from build123d import *

# Parameters (mm, degrees)
PAD_DEPTH            = 6.5
POCKET_DEPTH         = 6
SKETCH002_R          = 13.5
POCKET001_DEPTH      = 1
SKETCH003_W          = 5.4
SKETCH003_H          = 6.5
PAD001_DEPTH         = 3.5
POCKET002_DEPTH      = 10
SKETCH010_W          = 3.95
SKETCH010_H          = 6.5
PAD002_DEPTH         = 3.5
POCKET005_DEPTH      = 10
SKETCH014_R          = 20.45
SKETCH014_R_2        = 19.85
POCKET008_DEPTH      = 0.3
SKETCH015_R          = 2.2
SKETCH015_R_2        = 1.025
PAD003_DEPTH         = 2
POCKET009_DEPTH      = 4
POCKET010_DEPTH      = 4
PAD004_DEPTH         = 4
POCKET013_DEPTH      = 12.151
POCKET013_DEPTH_BACK = 36.251
SKETCH022_R          = 0.6
POCKET014_DEPTH      = 2
SKETCH023_R          = 0.6
POCKET015_DEPTH      = 2


with BuildPart() as part:
    # Sketch → Pad (new body)
    with BuildSketch(Plane.XY):
        with BuildLine():
            Line((-22.5019915649, 16), (-22.5019915649, -16))
            Line((-22.5019915649, -16), (-16.2858834578, -17.9))
            ThreePointArc((-16.2858834578, -17.9), (-0.4552796053, -24.1957169863), (15.6009615088, -18.5))
            Line((15.6009615088, -18.5), (24.5395016581, -17.45))
            Line((24.5395016581, 17.45), (24.5395016581, -17.45))
            Line((15.6009615088, 18.5), (24.5395016581, 17.45))
            ThreePointArc((15.6009615088, 18.5), (-0.4552796053, 24.1957169863), (-16.2858834578, 17.9))
            Line((-22.5019915649, 16), (-16.2858834578, 17.9))
        make_face()
    extrude(amount=PAD_DEPTH)

    # Sketch001 → Pocket (cut)
    with BuildSketch(Plane.XY):
        with BuildLine():
            Line((-14.8539557021, 16.9), (-21.2122180433, 15.55))
            Line((-21.2122180433, 15.55), (-21.2122180433, -15.55))
            Line((-21.2122180433, -15.55), (-14.8539557021, -16.9))
            ThreePointArc((-14.8539557021, -16.9), (-0.0760301383, -22.4998715423), (14.739402973, -17))
            Line((14.739402973, -17), (23.6191552218, -16.4))
            Line((23.6191552218, 16.4), (23.6191552218, -16.4))
            Line((14.739402973, 17), (23.6191552218, 16.4))
            ThreePointArc((14.739402973, 17), (-0.0760301383, 22.4998715423), (-14.8539557021, 16.9))
        make_face()
    extrude(amount=POCKET_DEPTH, mode=Mode.SUBTRACT)

    # Sketch002 (on Face19 of Pocket) → Pocket001 (cut)
    with BuildSketch(Plane(origin=(0, 0, 6), x_dir=(1, 0, 0), z_dir=(0, 0, -1))):
        Circle(SKETCH002_R)
    extrude(amount=-POCKET001_DEPTH, mode=Mode.SUBTRACT)

    # Sketch003 (on Face7 of Pad) → Pad001 (join)
    with BuildSketch(Plane.YZ.offset(24.5395016581)):
        with Locations((-14.75, 3.25)):
            Rectangle(SKETCH003_W, SKETCH003_H)
        with Locations((14.75, 3.25)):
            Rectangle(SKETCH003_W, SKETCH003_H)
    extrude(amount=PAD001_DEPTH)

    # Sketch006 (on Face22 of Pad001) → Pocket002 (cut)
    with BuildSketch(Plane.XY.offset(6.5)):
        with BuildLine():
            ThreePointArc((24.5395016581, 17.45), (26.1592830786, 16.2095505764), (28.0395016581, 15.4176006311))
            Line((28.0395016581, 17.45), (28.0395016581, 15.4176006311))
            Line((28.0395016581, 17.45), (24.5395016581, 17.45))
        make_face()
        with BuildLine():
            ThreePointArc((28.0395016581, -15.4176006311), (26.1592830786, -16.2095505765), (24.5395016581, -17.4500000001))
            Line((28.0395016581, -17.45), (24.5395016581, -17.45))
            Line((28.0395016581, -15.4176006311), (28.0395016581, -17.45))
        make_face()
    extrude(amount=-POCKET002_DEPTH, mode=Mode.SUBTRACT)

    # Sketch010 (on Face3 of Pad) → Pad002 (join)
    with BuildSketch(Plane(origin=(-22.5019915649, 0, 0), x_dir=(0, -1, 0), z_dir=(-1, 0, 0))):
        with Locations((-14.025, 3.25)):
            Rectangle(SKETCH010_W, SKETCH010_H)
        with Locations((14.025, 3.25)):
            Rectangle(SKETCH010_W, SKETCH010_H)
    extrude(amount=PAD002_DEPTH)

    # Sketch011 (on Face28 of Pad002) → Pocket005 (cut)
    with BuildSketch(Plane.XY.offset(6.5)):
        Polygon((-26.0019915649, 16), (-22.5019915649, 16), (-26.0019915649, 14.5), align=None)
        Polygon((-22.5019915649, -16), (-26.0019915649, -14.5), (-26.0019915649, -16), align=None)
    extrude(amount=-POCKET005_DEPTH, mode=Mode.SUBTRACT)

    # Sketch014 (on Face10 of Pad) → Pocket008 (cut)
    with BuildSketch(Plane.XY.offset(6.5)):
        Circle(SKETCH014_R)
        Circle(SKETCH014_R_2, mode=Mode.SUBTRACT)
    extrude(amount=-POCKET008_DEPTH, mode=Mode.SUBTRACT)

    # Sketch015 (on Face19 of Pocket) → Pad003 (join)
    with BuildSketch(Plane(origin=(0, 0, 6), x_dir=(1, 0, 0), z_dir=(0, 0, -1))):
        with Locations((-18.42, 13.32)):
            Circle(SKETCH015_R)
        with Locations((-18.42, 13.32)):
            Circle(SKETCH015_R_2, mode=Mode.SUBTRACT)
        with Locations((7.27, 18.56)):
            Circle(SKETCH015_R)
        with Locations((7.27, 18.56)):
            Circle(SKETCH015_R_2, mode=Mode.SUBTRACT)
        with Locations((5.37, -19.79)):
            Circle(SKETCH015_R)
        with Locations((5.37, -19.79)):
            Circle(SKETCH015_R_2, mode=Mode.SUBTRACT)
        with Locations((-18.42, -13.32)):
            Circle(SKETCH015_R)
        with Locations((-18.42, -13.32)):
            Circle(SKETCH015_R_2, mode=Mode.SUBTRACT)
    extrude(amount=PAD003_DEPTH)

    # Sketch016 (on Face4 of Pocket) → Pocket009 (cut)
    with BuildSketch(Plane(origin=(0, 0, 0), x_dir=(1, 0, 0), z_dir=(0, 0, -1))):
        with BuildLine():
            Line((-4.9992330338, 23.6779996848), (-5.0007669662, 21.9372361465))
            ThreePointArc((5.0007669662, 21.9372361465), (0, 22.5), (-5.0007669662, 21.9372361465))
            Line((5.0007669662, 23.6776757675), (5.0007669662, 21.9372361465))
            ThreePointArc((5.0007669662, 23.6776757675), (0.00078388, 24.1999999873), (-4.9992330338, 23.6779996848))
        make_face()
    extrude(amount=-POCKET009_DEPTH, mode=Mode.SUBTRACT)

    # Sketch017 (on Face4 of Pocket) → Pocket010 (cut)
    with BuildSketch(Plane(origin=(0, 0, 0), x_dir=(1, 0, 0), z_dir=(0, 0, -1))):
        with BuildLine():
            ThreePointArc((-3.2541322314, -22.2634369184), (0, -22.5), (3.2541322314, -22.2634369184))
            Line((3.2541322314, -22.2634369184), (3.5, -23.9455632634))
            ThreePointArc((-3.5, -23.9455632634), (0, -24.2), (3.5, -23.9455632634))
            Line((-3.2541322314, -22.2634369184), (-3.5, -23.9455632634))
        make_face()
        with BuildLine():
            ThreePointArc((-13.9498796389, -17.6536358312), (-11.25, -19.4855715851), (-8.3135572795, -20.9077680626))
            Line((-8.3135572795, -20.9077680626), (-8.9416927184, -22.487466094))
            ThreePointArc((-15.0038705449, -18.987466094), (-12.1, -20.9578147716), (-8.9416927184, -22.487466094))
            Line((-13.9498796389, -17.6536358312), (-15.0038705449, -18.987466094))
        make_face()
        with BuildLine():
            ThreePointArc((8.3135572795, -20.9077680626), (11.25, -19.4855715851), (13.9498796389, -17.6536358312))
            Line((13.9498796389, -17.6536358312), (15.0038705449, -18.987466094))
            ThreePointArc((8.9416927184, -22.487466094), (12.1, -20.9578147716), (15.0038705449, -18.987466094))
            Line((8.3135572795, -20.9077680626), (8.9416927184, -22.487466094))
        make_face()
    extrude(amount=-POCKET010_DEPTH, mode=Mode.SUBTRACT)

    # Sketch018 (on Face8 of Pocket005) → Pad004 (join)
    with BuildSketch(Plane(origin=(0, 0, 0), x_dir=(1, 0, 0), z_dir=(0, 0, -1))):
        Polygon((-26.0019915649, 14.5), (-26.0019915649, 12.05), (-22.5019915649, 12.05), (-22.5019915649, 16), align=None)
        Polygon((-26.0019915649, -12.05), (-22.5019915649, -12.05), (-22.5019915649, -16), (-26.0019915649, -14.5), align=None)
        with BuildLine():
            Line((24.5395016581, 17.4500000001), (24.5395016581, 12.05))
            Line((28.0395016581, 12.05), (24.5395016581, 12.05))
            Line((28.0395016581, 15.4176006311), (28.0395016581, 12.05))
            ThreePointArc((24.5395016581, 17.4500000001), (26.1592830786, 16.2095505765), (28.0395016581, 15.4176006311))
        make_face()
        with BuildLine():
            Line((24.5395016581, -12.05), (24.5395016581, -17.45))
            ThreePointArc((28.0395016581, -15.4176006311), (26.1592830786, -16.2095505764), (24.5395016581, -17.45))
            Line((28.0395016581, -12.05), (28.0395016581, -15.4176006311))
            Line((24.5395016581, -12.05), (28.0395016581, -12.05))
        make_face()
    extrude(amount=PAD004_DEPTH)

    # Sketch021 (on Face50 of Pad004) → Pocket013 (cut, two sides)
    with BuildSketch(Plane(origin=(0, -12.05, 0), x_dir=(-1, 0, 0), z_dir=(0, 1, 0))) as pocket013_sk:
        with BuildLine():
            Line((-24.8620157143, 6.5), (-28.0395016581, 6.5))
            Line((-28.0395016581, 6.5), (-28.0395016581, 2.1))
            ThreePointArc((-24.8620157143, 6.5), (-26.8441838951, 4.5841143344), (-28.0395016581, 2.1))
        make_face()
        with BuildLine():
            ThreePointArc((-25.9995016581, -4), (-25.0260575173, -3.5134441408), (-24.5395016581, -2.54))
            Line((-24.5395016581, -4), (-24.5395016581, -2.54))
            Line((-24.5395016581, -4), (-25.9995016581, -4))
        make_face()
        with BuildLine():
            Line((22.5019915649, -4), (22.5019915649, -2.54))
            ThreePointArc((22.5019915649, -2.54), (22.9885474241, -3.5134441408), (23.9619915649, -4))
            Line((22.5019915649, -4), (23.9619915649, -4))
        make_face()
        with BuildLine():
            Line((26.0019915649, 6.5), (26.0019915649, 2.1))
            ThreePointArc((26.0019915649, 2.1), (24.806673802, 4.5841143344), (22.8245056212, 6.5))
            Line((26.0019915649, 6.5), (22.8245056212, 6.5))
        make_face()
    extrude(amount=-POCKET013_DEPTH, mode=Mode.SUBTRACT)
    extrude(pocket013_sk.sketch, amount=POCKET013_DEPTH_BACK, mode=Mode.SUBTRACT)

    # Sketch022 (on Face66 of Pocket013) → Pocket014 (cut)
    with BuildSketch(Plane.XZ.offset(-12.05)):
        with Locations((-24.7019915649, -2.7)):
            Circle(SKETCH022_R)
        with Locations((26.7395016581, -2.7)):
            Circle(SKETCH022_R)
    extrude(amount=-POCKET014_DEPTH, mode=Mode.SUBTRACT)

    # Sketch023 (on Face49 of Pocket014) → Pocket015 (cut)
    with BuildSketch(Plane(origin=(0, -12.05, 0), x_dir=(-1, 0, 0), z_dir=(0, 1, 0))):
        with Locations((-26.7395016581, -2.7)):
            Circle(SKETCH023_R)
        with Locations((24.7019915649, -2.7)):
            Circle(SKETCH023_R)
    extrude(amount=-POCKET015_DEPTH, mode=Mode.SUBTRACT)


solid = part.part
Input: part model. Units: mm. Frame: model coordinates. A direction names the side the tool comes from. Give positions to 0.01 mm unless a question says otherwise; leave off trailing zeros. Order: outer loops, then holes, each group sorted by start corner. A loop starts at its lowest first (then second) coordinate and runs counter-clockwise, first axis right, second up. Notation, with made-up numbers: (-10.5, 68) -> (47.5, 68) arc R20 ccw to (47.5, 106) -> close; hole circle Ø4 at (88, 5). An arc over 180 degrees is marked (long way). Use one line per item in the form item = value.
1) Reachability of faces 1 (the cylindrical face through (-19.444, 13.275, 5.014)), 2 (the flat face through (-3.375, 23.093, 1.972)), 3 (the flat face through (8.623, 21.687, 1.972)) from +Z, -Z, +X, -X, +Y, -Y: full face, straight path, thin tool, end or side. Return the list, or none.
Response values:
face_1 = -Z
face_2 = -Z, +Y
face_3 = -Z, +X
2) Section C-C, the plane z = 1. Count the separate pieces of the cut face and the enclosed holes in it, and give its area (3 significant figures).
Response values:
separate_pieces = 4
enclosed_holes = 0
area = 224 mm^2
3) First-contact query: pin 1 Ø1.2 at (x, y) = (5.37, 19.79) entering from -Z; pin 2 Ø1.4 at (x, z) = (-24.7, -2.7) entering from +Y; pin 3 Ø0.9 at (y, z) = (-22.5, 2.5) entering from -X. Flat tips, straight axial feed; report the tip coordinate or a pass-through.
Response values:
pin_1 = 6
pin_2 = 15.36
pin_3 = -9.97
4) Section A-A, the plane x = 0. Return loops of the section in (y, z).
Response values:
outline = (-24.2, 4) -> (-22.5, 4) -> (-22.5, 6) -> (-13.5, 6) -> (-13.5, 6.5) -> (-19.85, 6.5) -> (-19.85, 6.2) -> (-20.45, 6.2) -> (-20.45, 6.5) -> (-24.2, 6.5) -> close; (13.5, 6) -> (22.5, 6) -> (22.5, 4) -> (24.2, 4) -> (24.2, 6.5) -> (20.45, 6.5) -> (20.45, 6.2) -> (19.85, 6.2) -> (19.85, 6.5) -> (13.5, 6.5) -> close
5) Section B-B, the plane y = 0. Return loops of the section in (x, z), and give its area (3 significant figures).
Response values:
outline = (-22.5, 0) -> (-21.21, 0) -> (-21.21, 6) -> (-13.5, 6) -> (-13.5, 6.5) -> (-19.85, 6.5) -> (-19.85, 6.2) -> (-20.45, 6.2) -> (-20.45, 6.5) -> (-22.5, 6.5) -> close; (13.5, 6) -> (23.62, 6) -> (23.62, 0) -> (24.54, 0) -> (24.54, 6.5) -> (20.45, 6.5) -> (20.45, 6.2) -> (19.85, 6.2) -> (19.85, 6.5) -> (13.5, 6.5) -> close
area = 22.9 mm^2
6) Line query: probe 1 along X at (y, z) = (8, 0.5); probe 2 along X at (y, z) = (14, 5); probe 3 along Y at (x, z) = (7.27, 5.55) (3 decimals). Output: solid intervals per line, ascending.
Response values:
probe_1 = -22.5 to -21.21, 23.62 to 24.54
probe_2 = -24.48 to -21.21, -20.51 to -19.19, -17.65 to -16.33, 23.62 to 26.52
probe_3 = -23.082 to -21.293, -20.76 to -19.585, -17.535 to -16.36, 18.681 to 20.899, 21.293 to 23.082
7) Mould query, pull axis Y, two halves, no side actions, for faces 4 (the flat face through (-19.437, -16.937, 3.204)), 5 (the flat face through (27, 14.05, -3)), 6 (the flat face through (24.54, 15, -1)). Classes: pulls with the +Y half, pulls with the -Y half, needs draft (parallel to the pull), parting line crosses it, or undercut.
Response values:
face_4 = pulls with the -Y half
face_5 = undercut
face_6 = needs draft
